For this review, take the finished solid that the model builds, in its own axes (mm). Face numbers are marked on the shaded views. A direction names the side the tool comes from. Round coordinates to 2 decimals unless told otherwise and drop trailing zeros. Write each loop counter-clockwise with the first axis right and the second up, starting at its lowest first coordinate (ties: lowest second). Pieces come first, ordered by that corner, then holes. Notation, with made-up numbers: (22, 27.25) -> (32, 27.25) arc R27 cw to (32, 58.25) -> close; hole circle Ø3 at (62.5, 69.5). An arc over 180 degrees is marked (long way). Answer in a Markdown table with one row per item.
from build123d import *

# Parameters (mm, degrees)
F0_R     = 14
F1_DEPTH = 40
F2_R     = 4.733674
F2_R_2   = 5.5
F3_DEPTH = 25


with BuildPart() as f1:
    # F0 (on Front) → F1 (new body)
    with BuildSketch(Plane.XZ):
        with BuildLine():
            Line((-43.805312, -8.794249), (-43.805312, -23.794249))
            Line((-43.805312, -23.794249), (66.194688, -23.794249))
            Line((66.194688, -23.794249), (66.194688, -8.794249))
            Line((66.194688, -8.794249), (36.194688, -8.794249))
            Line((36.194688, -8.794249), (36.194688, 16.205751))
            ThreePointArc((36.194688, 16.205751), (11.194688, 41.205751), (-13.805312, 16.205751))
            Line((-13.805312, 16.205751), (-13.805312, -8.794249))
            Line((-13.805312, -8.794249), (-43.805312, -8.794249))
        make_face()
        with Locations((11.194688, 16.205751)):
            Circle(F0_R, mode=Mode.SUBTRACT)
    extrude(amount=F1_DEPTH)

    # F2 (on Top) → F3 (cut)
    with BuildSketch(Plane.XY):
        with Locations((-28.817502, -20)):
            Circle(F2_R)
        with Locations((51.097777, -19.957691)):
            Circle(F2_R_2)
    extrude(amount=-F3_DEPTH, mode=Mode.SUBTRACT)


solid = f1.part
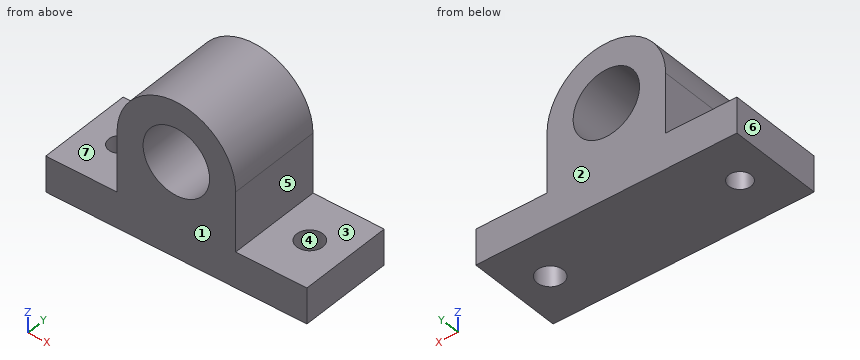
1) Clearance check with flat-ended pins moving along their axes: pin 1 Ø20 at (y, z) = (-10, 6.5) entering from +X; pin 2 Ø12 at (x, y) = (48.5, -10) entering from +Z; pin 3 Ø4 at (y, z) = (-10.5, 25) entering from -X. State where each tip first meets the part, or that it passes through.
Solved:
| item | result |
|---|---|
| pin 1 | x = 36.19 |
| pin 2 | z = -8.79 |
| pin 3 | x = -12.86 |
2) Consider section A-A on y = -22.5. State the section outline as (x, z) points.
Solved:
| item | result |
|---|---|
| outline | (-43.81, -23.79) -> (-32.84, -23.79) -> (-32.84, -8.79) -> (-43.81, -8.79) -> close; (-24.8, -23.79) -> (46.22, -23.79) -> (46.22, -8.79) -> (36.19, -8.79) -> (36.19, 16.21) arc R25 ccw to (-13.81, 16.21) -> (-13.81, -8.79) -> (-24.8, -8.79) -> close; (55.97, -23.79) -> (66.19, -23.79) -> (66.19, -8.79) -> (55.97, -8.79) -> close; hole circle Ø28 at (11.19, 16.21) |
3) For the marked faces 5, 6 and 7, list the 3-axis set-ups (+Z, -Z, +X, -X, +Y, -Y) from which the entire face can be reached by the end or side of a thin tool; tool diameter is ignored.
Solved:
| item | result |
|---|---|
| face 5 | +Z, +X, +Y, -Y |
| face 6 | +Z, -Z, -X, +Y, -Y |
| face 7 | +Z, -X, +Y, -Y |
4) Consider section B-B on x = 7. State the section outline as (y, z) points, then the cut area to 3 significant figures.
Solved:
| item | result |
|---|---|
| outline | (-40, -23.79) -> (0, -23.79) -> (0, 2.85) -> (-40, 2.85) -> close; (-40, 29.56) -> (0, 29.56) -> (0, 40.85) -> (-40, 40.85) -> close |
| area | 1,520 mm² |
5) Mouldability with a two-part tool opening along Y and no side actions: class the marked faces 1, 2, 3 and 4 as pulls with the +Y half, pulls with the -Y half, needs draft (parallel to the pull), parting line crosses it, or undercut.
Solved:
| item | result |
|---|---|
| face 1 | pulls with the -Y half |
| face 2 | pulls with the +Y half |
| face 3 | needs draft |
| face 4 | undercut |
6) Consider section C-C on z = 28. State the section outline as (x, y) points.
Solved:
| item | result |
|---|---|
| outline | (-10.85, -40) -> (3.65, -40) -> (3.65, 0) -> (-10.85, 0) -> close; (18.74, -40) -> (33.24, -40) -> (33.24, 0) -> (18.74, 0) -> close |
7) Consider section D-D on y = -32. State the section outline as (x, z) points.
Solved:
| item | result |
|---|---|
| outline | (-43.81, -23.79) -> (66.19, -23.79) -> (66.19, -8.79) -> (36.19, -8.79) -> (36.19, 16.21) arc R25 ccw to (-13.81, 16.21) -> (-13.81, -8.79) -> (-43.81, -8.79) -> close; hole circle Ø28 at (11.19, 16.21) |
8) For line 1 (Z direction, x = -35.5, y = -31); line 2 (X direction, y = -33, z = -0.5); line 3 (X direction, y = -26.5, z = 26.5), list the stretches that pass through material, from the lowest coordinate up. Write a range as [from, to].
Solved:
| item | result |
|---|---|
| line 1 | [-23.79, -8.79] |
| line 2 | [-13.81, 36.19] |
| line 3 | [-11.59, 1.71], [20.68, 33.98] |
